from build123d import *

# Parameters (mm, degrees)
F0_W        = 6.35
F0_H        = 12.7
F1_DEPTH    = 7.62
F3_DEPTH    = 6.35
F4_T1_DEPTH = 28.3769794946
F5_R        = 0.762


# Not quite as in the source:
# - a fillet or chamfer that OpenCascade refuses, or shapes differently, is made with other operations: its cross-section is extruded or revolved along the edge and cut away or added
# - a feature names something its author has since deleted; it is built from what else it names


with BuildPart() as f1:
    # F0 (on Top) → F1 (new body)
    with BuildSketch(Plane.XY):
        with Locations((-47.625, -6.35)):
            Rectangle(F0_W, F0_H)
    extrude(amount=F1_DEPTH)

    # F2 (on face) → F3 (cut)
    with BuildSketch(Plane.XY.offset(7.62)):
        with BuildLine():
            ThreePointArc((-45.72, -6.223), (-47.625, -4.318), (-49.53, -6.223))
            Line((-49.53, -6.223), (-49.53, -9.525))
            ThreePointArc((-49.53, -9.525), (-47.625, -11.43), (-45.72, -9.525))
            Line((-45.72, -9.525), (-45.72, -6.223))
        make_face()
    extrude(amount=-F3_DEPTH, mode=Mode.SUBTRACT)

    # F4: chamfer of 3.048 on 2 edges, made by hand

    # F4_s2 → F4_t1 (cut)
    with BuildSketch(Plane.XZ.offset(-7.8384897473)):
        Polygon((-50.8, 4.572), (-47.752, 7.62), (-50.8, 7.62), align=None)
        Polygon((-44.45, 4.572), (-47.498, 7.62), (-44.45, 7.62), align=None)
    extrude(amount=F4_T1_DEPTH, mode=Mode.SUBTRACT)

    # F5
    f5_edges = [f1.edges().sort_by_distance(p)[0] for p in [
        (-50.8, -6.35, 0),
        (-44.45, -6.35, 0),
    ]]
    fillet(f5_edges, radius=F5_R)


solid = f1.part
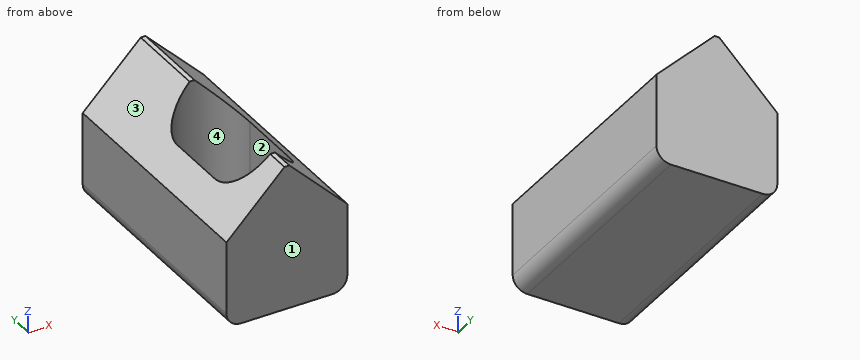
Design review of the part built by this model. Coordinates are the model's own, in mm. Face numbers are marked on the shaded views. Round coordinates to 2 decimals unless told otherwise and drop trailing zeros. Write each loop counter-clockwise with the first axis right and the second up, starting at its lowest first coordinate (ties: lowest second). Pieces come first, ordered by that corner, then holes. Notation, with made-up numbers: (40, 81.5) -> (67, 81.5) arc R14 cw to (67, 100.5) -> close; hole circle Ø4 at (3, -33.5). An arc over 180 degrees is marked (long way). One line per item, written item: value. Start each with the question number.
Q1. Add section C-C (z = 2). Give the boundary of the cut face in (x, y) (3 decimals).
Q2. Add section D-D (x = -48). Give the boundary of the cut face in (y, z).
Q3. Add section A-A (z = 7). Give the boundary of the cut face in (x, y) (3 decimals).
Q4. To check wall thickness, follow probe 1 along X at (y, z) = (-9, 1.75); probe 2 along Z at (x, y) = (-46.5, -5.75); probe 3 along Y at (x, z) = (-46.5, 4.75). State the ranges of each line that lie inside material, in increasing order.
Q5. The part is to be moulded in two halves that separate along Y. For the marked faces 1, 2, 3 and 4, say which applies: pulls with the +Y half, pulls with the -Y half, needs draft (parallel to the pull), parting line crosses it, or undercut.
Q6. Add section B-B (y = -2). Give the boundary of the cut face in (x, z), then the cut area to 3 significant figures.
Response:
1. outline: (-50.8, -12.7) -> (-44.45, -12.7) -> (-44.45, 0) -> (-50.8, 0) -> close; hole (-49.53, -9.525) arc R1.905 ccw to (-45.72, -9.525) -> (-45.72, -6.223) arc R1.905 ccw to (-49.53, -6.223) -> close
2. outline: (-12.7, 0) -> (0, 0) -> (0, 7.37) -> (-4.36, 7.37) -> (-4.36, 1.27) -> (-11.39, 1.27) -> (-11.39, 7.37) -> (-12.7, 7.37) -> close
3. outline: (-48.372, -12.7) -> (-46.878, -12.7) -> (-46.878, -11.277) arc R1.905 cw to (-48.372, -11.277) -> close; (-48.372, -4.471) arc R1.905 cw to (-46.878, -4.471) -> (-46.878, 0) -> (-48.372, 0) -> close
4. probe 1: x = -50.8 to -49.53, -45.72 to -44.45
4. probe 2: z = 0 to 1.27
4. probe 3: y = -12.7 to -11.06, -4.69 to 0
5. face 1: pulls with the -Y half
5. face 2: undercut
5. face 3: needs draft
5. face 4: undercut
6. outline: (-50.8, 0.76) arc R0.76 ccw to (-50.04, 0) -> (-45.21, 0) arc R0.76 ccw to (-44.45, 0.76) -> (-44.45, 4.57) -> (-47.5, 7.62) -> (-47.75, 7.62) -> (-50.8, 4.57) -> close
6. area: 38.8 mm^2
